Verification items for the finished model (mm, model axes). A direction names the side the tool comes from. Give positions to 0.01 mm unless a question says otherwise; leave off trailing zeros. Order: outer loops, then holes, each group sorted by start corner. A loop starts at its lowest first (then second) coordinate and runs counter-clockwise, first axis right, second up. Notation, with made-up numbers: (-12, -24.5) -> (-2, -24.5) arc R15 ccw to (-2, -17.5) -> close; hole circle Ø3 at (35, -28). An arc over 180 degrees is marked (long way). Return JSON: item names as keys, results as strings. Group by question number.
(1) Thickness scan on line 1 along Z through (x, y) = (0, 7.5); line 2 along Z through (x, y) = (-10, -2.5); line 3 along X through (y, z) = (9.25, 5). Record the ranges inside material, lowest first.
(2) Cross-section at A-A on x = 0. Enter the section's corners in (y, z).
(3) Depth check by flat-ended pin: pin 1 Ø5 at (x, z) = (15.475, -4.875) entering from -Y; pin 2 Ø12 at (y, z) = (5, -26.5) entering from +X; pin 3 Ø6 at (x, y) = (6, -8) entering from +Z; pin 4 Ø5 at (x, z) = (-37, -17) entering from -Y. Enter the tip coordinate at first touch or a pass-through.
(4) Release check for a two-part mould opening along Z. For faces 1 (the face through (-13.77, 6.26, 61.99)), 2 (the face through (-1, 12.7, 13)), 3 (the face through (-44.743, 6.261, 1.907)), 4 (the face through (-6, -6, 17.78)) record: pulls with the +Z half, pulls with the -Z half, needs draft (parallel to the pull), parting line crosses it, or undercut.
(5) Tool access check on faces 5 (the face through (-33, -1.45, 0)), 6 (the face through (-37.464, -5.724, 0.259)), 7 (the face through (11.684, -6, 0)), 8 (the face through (21.59, -6, 0)). Record the directions out of +Z, -Z, +X, -X, +Y, -Y that give a thin tool (end or side, any length) a straight path to the whole face; none if there is none.
(6) Cross-section at C-C on y = 8.5. Enter the section's corners in (x, z), then the cut area to 3 significant figures.
(7) Cross-section at B-B on z = 0. Enter the section's corners in (x, y) (3 decimals), then the cut area to 3 significant figures.
(8) Cross-section at D-D on x = -50.8. Enter the section's corners in (y, z), then the cut area to 3 significant figures.
from build123d import *

# Parameters (mm, degrees)
SKETCH2_R           = 63.5
BOSS_EXTRUDE1_DEPTH = 12.7
SKETCH3_R           = 6.35
CUT_EXTRUDE1_DEPTH  = 13.7
SKETCH6_W           = 55.88
SKETCH6_H           = 20.32
CUT_EXTRUDE3_DEPTH  = 27.686
SKETCH8_W           = 60.96
SKETCH8_H           = 35.56
SKETCH8_W_2         = 55.88
SKETCH8_H_2         = 20.32
BOSS_EXTRUDE2_DEPTH = 1.45
SKETCH9_W           = 60.96
SKETCH9_H           = 35.56
SKETCH9_R           = 2.105780523
SKETCH9_W_2         = 41.148
SKETCH9_H_2         = 20.32
BOSS_EXTRUDE3_DEPTH = 10.16
SKETCH11_R          = 63.5
SKETCH11_R_2        = 37.465
CUT_EXTRUDE5_DEPTH  = 12.61


with BuildPart() as part:
    # Sketch2 → Boss-Extrude1 (new body)
    with BuildSketch(Plane(origin=(0, 0, 0), x_dir=(1, 0, 0), z_dir=(0, 1, 0))):
        Circle(SKETCH2_R)
    extrude(amount=BOSS_EXTRUDE1_DEPTH)

    # Sketch3 → Cut-Extrude1 (cut, through all)
    with BuildSketch(Plane.XZ):
        with Locations((0, 50.8)):
            Circle(SKETCH3_R)
        with Locations((-50.8, 0)):
            Circle(SKETCH3_R)
        with Locations((0, -50.8)):
            Circle(SKETCH3_R)
        with Locations((50.8, 0)):
            Circle(SKETCH3_R)
    extrude(amount=-CUT_EXTRUDE1_DEPTH, mode=Mode.SUBTRACT)

    # Sketch6 → Cut-Extrude3 (cut)
    with BuildSketch(Plane.XZ):
        with Locations((-8.89, 0)):
            Rectangle(SKETCH6_W, SKETCH6_H)
    extrude(amount=-CUT_EXTRUDE3_DEPTH, mode=Mode.SUBTRACT)

    # Sketch8 → Boss-Extrude2 (add)
    with BuildSketch(Plane.XZ):
        with Locations((-8.89, 0)):
            Rectangle(SKETCH8_W, SKETCH8_H)
        with Locations((-8.89, 0)):
            Rectangle(SKETCH8_W_2, SKETCH8_H_2, mode=Mode.SUBTRACT)
    extrude(amount=BOSS_EXTRUDE2_DEPTH)

    # Sketch9 → Boss-Extrude3 (add)
    with BuildSketch(Plane.XZ.offset(1.45)):
        with Locations((-8.89, 0)):
            Rectangle(SKETCH9_W, SKETCH9_H)
        with Locations((-33.125, 4.875)):
            Circle(SKETCH9_R, mode=Mode.SUBTRACT)
        with Locations((-33.125, -4.875)):
            Circle(SKETCH9_R, mode=Mode.SUBTRACT)
        with Locations((15.475, 4.875)):
            Circle(SKETCH9_R, mode=Mode.SUBTRACT)
        with Locations((15.475, -4.875)):
            Circle(SKETCH9_R, mode=Mode.SUBTRACT)
        with Locations((-8.89, 0)):
            Rectangle(SKETCH9_W_2, SKETCH9_H_2, mode=Mode.SUBTRACT)
    extrude(amount=BOSS_EXTRUDE3_DEPTH)

    # Sketch11 → Cut-Extrude5 (cut, through all)
    with BuildSketch(Plane.XZ):
        Circle(SKETCH11_R)
        Circle(SKETCH11_R_2, mode=Mode.SUBTRACT)
    extrude(amount=CUT_EXTRUDE5_DEPTH, mode=Mode.SUBTRACT)


solid = part.part
Verdict:
{
 "1": {"line 1": "-63.5 to -57.15, -44.45 to -10.16, 10.16 to 44.45, 57.15 to 63.5", "line 2": "-17.78 to -10.16, 10.16 to 17.78", "line 3": "-63.3 to -54.71, -46.89 to -36.83, 19.05 to 46.89, 54.71 to 63.3"},
 "2": {"outline": "(-11.61, -17.78) -> (0, -17.78) -> (0, -44.45) -> (12.7, -44.45) -> (12.7, -10.16) -> (-11.61, -10.16) -> close; (-11.61, 10.16) -> (12.7, 10.16) -> (12.7, 44.45) -> (0, 44.45) -> (0, 17.78) -> (-11.61, 17.78) -> close; (0, -63.5) -> (12.7, -63.5) -> (12.7, -57.15) -> (0, -57.15) -> close; (0, 57.15) -> (12.7, 57.15) -> (12.7, 63.5) -> (0, 63.5) -> close"},
 "3": {"pin 1": "y = -11.61", "pin 2": "x = 60.1", "pin 3": "z = 17.78", "pin 4": "y = 0"},
 "4": {"face 1": "parting line crosses it", "face 2": "needs draft", "face 3": "undercut", "face 4": "pulls with the +Z half"},
 "5": {"face 5": "+Y", "face 6": "-X, -Y", "face 7": "+Y, -Y", "face 8": "+Z, -Z, +X, -Y"},
 "6": {"outline": "circle Ø127 at (0, 0); hole circle Ø12.7 at (-50.8, 0); hole (-36.83, -10.16) -> (19.05, -10.16) -> (19.05, 10.16) -> (-36.83, 10.16) -> close; hole circle Ø12.7 at (0, -50.8); hole circle Ø12.7 at (0, 50.8); hole circle Ø12.7 at (50.8, 0)", "area": "11,000 mm²"},
 "7": {"outline": "(-63.5, 0) -> (-57.15, 0) -> (-57.15, 12.7) -> (-63.5, 12.7) -> close; (-44.45, 0) -> (-37.465, 0) -> (-37.465, -11.61) -> (-29.464, -11.61) -> (-29.464, -1.45) -> (-36.83, -1.45) -> (-36.83, 12.7) -> (-44.45, 12.7) -> close; (11.684, -11.61) -> (21.59, -11.61) -> (21.59, 0) -> (44.45, 0) -> (44.45, 12.7) -> (19.05, 12.7) -> (19.05, -1.45) -> (11.684, -1.45) -> close; (57.15, 0) -> (63.5, 0) -> (63.5, 12.7) -> (57.15, 12.7) -> close", "area": "767 mm²"},
 "8": {"outline": "(0, -38.1) -> (12.7, -38.1) -> (12.7, -6.35) -> (0, -6.35) -> close; (0, 6.35) -> (12.7, 6.35) -> (12.7, 38.1) -> (0, 38.1) -> close", "area": "806 mm²"}
}
